Autodesk Fusion 360 part; units mm, degrees
sketch "Sketch1" plane through (0, 0, 0) normal (0, 1, 0) x (1, 0, 0)
  circle A0 centre (0, 0) radius 10.5
  dimension "d1" = 21
extrude "Extrude1" add sketch "Sketch1" along normal blind 17
sketch "Sketch2" plane through (0, 0, 0) normal (0, -1, 0) x (1, 0, 0)
  circle A0 centre (0, 0) radius 10.5
  circle A1 centre (0, 0) radius 13
  dimension "d4" = 26
extrude "Extrude2" add sketch "Sketch2" along normal blind 3 contours A0 | A1
sketch "Sketch3" plane through (0, 17, 0) normal (0, 1, 0) x (-1, 0, 0)
  circle A0 centre (0, 0) radius 10.5
  circle A1 centre (0, 0) radius 13
  dimension "d7" = 26
extrude "Extrude3" add sketch "Sketch3" along normal blind 3 contours A0 | A1
sketch "Sketch4" plane through (0, -3, 0) normal (0, -1, 0) x (1, 0, 0)
  circle A0 centre (0, 0) radius 13
  circle A1 centre (0, 0) radius 2.6
  dimension "d10" = 5.2
extrude "Extrude4" cut sketch "Sketch4" against normal blind 6 contours A1
extrude "Extrude5" cut sketch "Sketch4" against normal blind 23 contours A1
Check sheet for the modelled part. Datum: model origin and axes. Units: mm. A direction names the side the tool comes from. Give positions to 0.01 mm unless a question says otherwise; leave off trailing zeros. Loops run counter-clockwise (first coordinate to the right, second up) from the corner with the lowest first, then second, coordinate; pieces in that order, holes last. Notation, with made-up numbers: M 63,-21 L 93,-21 A3 cw 93,-16 Z; hole C -19,49 d4. An arc over 180 degrees is marked long. Answer in a Markdown table with one row per item.
1) Depth check by flat-ended pin: pin 1 (1 mm diameter, centred on x = 2.5, y = 15.5, fed in from +Z); pin 2 (6 mm diameter, centred on y = 5, z = 8.5, fed in from +X); pin 3 (10 mm diameter, centred on y = 1, z = 7.5, fed in from -X). Enter the tip coordinate at first touch or a pass-through.
Solutions:
| item | result |
|---|---|
| pin 1 | stops at z = 10.31 |
| pin 2 | stops at x = 8.94 |
| pin 3 | stops at x = -12.74 |
2) Tool access check on faces 4 (the face through (10, 8.4, 3.2)), 5 (the face through (-10.316, -1.479, 7.91)). Record the directions out of +Z, -Z, +X, -X, +Y, -Y that give a thin tool (end or side, any length) a straight path to the whole face; none if there is none.
Solutions:
| item | result |
|---|---|
| face 4 | none |
| face 5 | +Y, -Y |
3) Cross-section at C-C (y = 13.5). Enter the section's corners in (x, z), plus the area to 3 significant figures.
Solutions:
| item | result |
|---|---|
| outline | C 0,0 d21; hole C 0,0 d5.2 |
| area | 325 mm^2 |
4) Thickness scan on line 1 (Z direction, x = 0, y = 5.75); line 2 (Y direction, x = 10.75, z = -3.25); line 3 (X direction, y = 13.25, z = -1). Record the ranges inside material, lowest first.
Solutions:
| item | result |
|---|---|
| line 1 | z = -10.5 to -2.6, 2.6 to 10.5 |
| line 2 | y = -3 to 0, 17 to 20 |
| line 3 | x = -10.45 to -2.4, 2.4 to 10.45 |
5) Mould release check, pull along Y, two halves, no side actions. Record for faces 1 (the face through (-0.338, 8.339, 2.578)), 2 (the face through (-3, 20, 0)), 3 (the face through (9, 17, 6)): released by +Y, released by -Y, zero draft, split by the parting line, or undercut.
Solutions:
| item | result |
|---|---|
| face 1 | zero draft |
| face 2 | released by +Y |
| face 3 | undercut |
6) Cross-section at B-B (x = 0). Enter the section's corners in (y, z), plus the area to 3 significant figures.
Solutions:
| item | result |
|---|---|
| outline | M -3,-13 L 0,-13 L 0,-10.5 L 17,-10.5 L 17,-13 L 20,-13 L 20,-2.6 L -3,-2.6 Z; M -3,2.6 L 20,2.6 L 20,13 L 17,13 L 17,10.5 L 0,10.5 L 0,13 L -3,13 Z |
| area | 393 mm^2 |
7) Cross-section at A-A (z = 0). Enter the section's corners in (x, y).
Solutions:
| item | result |
|---|---|
| outline | M -13,-3 L -2.6,-3 L -2.6,20 L -13,20 L -13,17 L -10.5,17 L -10.5,0 L -13,0 Z; M 2.6,-3 L 13,-3 L 13,0 L 10.5,0 L 10.5,17 L 13,17 L 13,20 L 2.6,20 Z |
8) Cross-section at D-D (z = 5.5). Enter the section's corners in (x, y).
Solutions:
| item | result |
|---|---|
| outline | M -11.78,-3 L 11.78,-3 L 11.78,0 L 8.94,0 L 8.94,17 L 11.78,17 L 11.78,20 L -11.78,20 L -11.78,17 L -8.94,17 L -8.94,0 L -11.78,0 Z |
